Here's how the part is built. I have some questions about the finished solid (model axes, mm). A direction names the side the tool comes from. Coordinates: 2 decimals unless noted, no trailing zeros. Write each loop counter-clockwise with the first axis right and the second up, starting at its lowest first coordinate (ties: lowest second). Pieces come first, ordered by that corner, then holes. Notation, with made-up numbers: M -14.75,86.25 L 4.25,86.25 A16 cw 4.25,107.25 Z; hole C 58.5,80 d10. An arc over 180 degrees is marked long. Use one line per item in the form item = value. Start each with the question number.
1. Please list where these lines run through material, in increasing order: line 1 along Z through (x, y) = (15.75, 351.5); line 2 along Y through (x, z) = (7.75, 8.5). Write a range as [from, to].
2. Thinking about a two-plate mould opening in Z: for faces 3 (the face through (13, 201, 22.8)), 4 (the face through (2.8, 201, 13)), 5 (the face through (2, 0, 13)), 6 (the face through (13, 207, 25.6)), which applies, released by +Z, released by -Z, zero draft, split by the parting line, or undercut?
3. I want a section at A-A, the plane y = 253.5. List the corners of the cut face in (x, z) for me, plus the area to 3 significant figures.
4. I'm going to push flat-ended pins straight in: pin 1 Ø8 at (x, z) = (5.5, 7) entering from -Y; pin 2 Ø1.5 at (x, z) = (13.5, 7.5) entering from -Y. Where does each tip first touch, or does it pass through?
5. I want a section at B-B, the plane x = 16.25. List the corners of the cut face in (y, z) for me.
6. I want a section at C-C, the plane z = 17.25. List the corners of the cut face in (x, y) for me, plus the area to 3 significant figures.
7. On a 3-axis mill with a long thin cutter (end or side, diameter ignored), from which of +Z, -Z, +X, -X, +Y, -Y can I reach the whole of each face in a straight line? I mean faces 1 (the face through (13, 419.01, 13)), 2 (the face through (13, 408.5, 13)). Say none if no direction works.
from build123d import *

# Parameters (mm, degrees)
BOSS_EXTRUDE1_DEPTH = 419.01
SKETCH3_W           = 20
SKETCH3_H           = 20
CUT_EXTRUDE1_DEPTH  = 408.5


with BuildPart() as part:
    # Sketch1 → Boss-Extrude1 (new body)
    with BuildSketch(Plane(origin=(0, 0, 0), x_dir=(1, 0, 0), z_dir=(0, 1, 0))):
        with BuildLine():
            Line((2.8, 0), (22.8, 0))
            ThreePointArc((22.8, 0), (24.779898987, -0.820101013), (25.6, -2.8))
            Line((25.6, -2.8), (25.6, -22.8))
            ThreePointArc((25.6, -22.8), (24.779898987, -24.779898987), (22.8, -25.6))
            Line((22.8, -25.6), (2.8, -25.6))
            ThreePointArc((2.8, -25.6), (0.820101013, -24.779898987), (0, -22.8))
            Line((0, -22.8), (0, -2.8))
            ThreePointArc((0, -2.8), (0.820101013, -0.820101013), (2.8, 0))
        make_face()
    extrude(amount=BOSS_EXTRUDE1_DEPTH)

    # Sketch3 → Cut-Extrude1 (cut)
    with BuildSketch(Plane(origin=(0, 0, 0), x_dir=(-1, 0, 0), z_dir=(0, -1, 0))):
        with Locations((-12.8, -12.8)):
            Rectangle(SKETCH3_W, SKETCH3_H)
    extrude(amount=-CUT_EXTRUDE1_DEPTH, mode=Mode.SUBTRACT)


solid = part.part
Answer list:
q1.line_1 = [0, 2.8], [22.8, 25.6]
q1.line_2 = [408.5, 419.01]
q2.face_3 = undercut
q2.face_4 = undercut
q2.face_5 = zero draft
q2.face_6 = released by +Z
q3.outline = M 0,2.8 A2.8 ccw 2.8,0 L 22.8,0 A2.8 ccw 25.6,2.8 L 25.6,22.8 A2.8 ccw 22.8,25.6 L 2.8,25.6 A2.8 ccw 0,22.8 Z; hole M 2.8,2.8 L 22.8,2.8 L 22.8,22.8 L 2.8,22.8 Z
q3.area = 249 mm²
q4.pin_1 = 0
q4.pin_2 = 408.5
q5.outline = M 0,0 L 419.01,0 L 419.01,25.6 L 0,25.6 L 0,22.8 L 408.5,22.8 L 408.5,2.8 L 0,2.8 Z
q6.outline = M 0,0 L 2.8,0 L 2.8,408.5 L 22.8,408.5 L 22.8,0 L 25.6,0 L 25.6,419.01 L 0,419.01 Z
q6.area = 2,560 mm²
q7.face_1 = +Z, -Z, +X, -X, +Y
q7.face_2 = -Y
